```python
from build123d import *

# Parameters (mm, degrees)
SKETCH1_W           = 29
SKETCH1_H           = 42
BOSS_EXTRUDE1_DEPTH = 1.5
SKETCH2_W           = 11.5
SKETCH2_H           = 10
BOSS_EXTRUDE2_DEPTH = 7
SKETCH3_R           = 3
BOSS_EXTRUDE3_DEPTH = 18
SKETCH4_R           = 3
BOSS_EXTRUDE4_DEPTH = 8


with BuildPart() as part:
    # Sketch1 → Boss-Extrude1 (new body)
    with BuildSketch(Plane.XY):
        Rectangle(SKETCH1_W, SKETCH1_H)
    extrude(amount=BOSS_EXTRUDE1_DEPTH)

    # Sketch2 → Boss-Extrude2 (add)
    with BuildSketch(Plane.XY.offset(1.5)):
        with Locations((0, -3)):
            Rectangle(SKETCH2_W, SKETCH2_H)
    extrude(amount=BOSS_EXTRUDE2_DEPTH)

    # Sketch3 → Boss-Extrude3 (add)
    with BuildSketch(Plane.XY.offset(8.5)):
        with Locations((0, -3)):
            Circle(SKETCH3_R)
    extrude(amount=BOSS_EXTRUDE3_DEPTH)

    # Sketch4 → Boss-Extrude4 (add)
    with BuildSketch(Plane.XY.offset(1.5)):
        with Locations((11.5, -1)):
            Circle(SKETCH4_R)
    extrude(amount=BOSS_EXTRUDE4_DEPTH)


solid = part.part
```
Check sheet for the modelled part. Datum: model origin and axes. Units: mm. A direction names the side the tool comes from. Coordinates: 2 decimals unless noted, no trailing zeros. Loops run counter-clockwise (first coordinate to the right, second up) from the corner with the lowest first, then second, coordinate; pieces in that order, holes last.
1) Release check for a two-part mould opening along X. For faces 4 (the face through (-5.75, -3, 5)), 5 (the face through (11, -1, 9.5)), 6 (the face through (5.75, -3, 5)) record: released by +X, released by -X, zero draft, split by the parting line, or undercut.
2) Sectioned sample at A-A (z = 6.25). Record the boundary of the cut face in (x, y).
3) Sectioned sample at B-B (x = 0). Record the boundary of the cut face in (y, z), and give its area (3 significant figures).
4) Gauge pin test, flat ends, axial feed: pin 1 (10 mm diameter, centred on x = -0.5, z = 5, fed in from -Y); pin 2 (10 mm diameter, centred on y = -5, z = 10.5, fed in from -X); pin 3 (2 mm diameter, centred on x = 2.5, z = 13, fed in from +Y); pin 4 (3 mm diameter, centred on x = 3, z = 11.5, fed in from -Y). Record the tip position at first contact, or that the pin passes through.
5) Material ranges on probe 1 along Z at (x, y) = (2.5, -15); probe 2 along Y at (x, z) = (-5, 5.5); probe 3 along Y at (x, z) = (-2, 19.5), recorded low to high.
6) Sectioned sample at C-C (z = 14). Record the boundary of the cut face in (x, y).
7) Access from +Z, -Z, +X, -X, +Y, -Y to the whole of each face (thin tool, end or side, straight path). Record for faces 1 (the face through (0, -8, 5)), 2 (the face through (9.1, -2.8, 5.4)), 3 (the face through (0, 2, 5)).
8) Sectioned sample at D-D (y = 13.5). Record the boundary of the cut face in (x, z).
Check sheet entries:
1. face 4: released by -X
1. face 5: zero draft
1. face 6: undercut
2. outline: (-5.75, -8) - (5.75, -8) - (5.75, 2) - (-5.75, 2) - close; circle Ø6 at (11.5, -1)
3. outline: (-21, 0) - (21, 0) - (21, 1.5) - (2, 1.5) - (2, 8.5) - (0, 8.5) - (0, 26.5) - (-6, 26.5) - (-6, 8.5) - (-8, 8.5) - (-8, 1.5) - (-21, 1.5) - close
3. area: 241 mm2
4. pin 1: stops at y = -21
4. pin 2: stops at x = -5.75
4. pin 3: stops at y = -0.4
4. pin 4: stops at y = -5.6
5. probe 1: z = 0 to 1.5
5. probe 2: y = -8 to 2
5. probe 3: y = -5.24 to -0.76
6. outline: circle Ø6 at (0, -3)
7. face 1: +Z, +X, -X, -Y
7. face 2: +Z
7. face 3: +Z, +X, -X, +Y
8. outline: (-14.5, 0) - (14.5, 0) - (14.5, 1.5) - (-14.5, 1.5) - close
